For this review, take the finished solid that the model builds, in its own axes (mm). A direction names the side the tool comes from. Round coordinates to 2 decimals unless told otherwise and drop trailing zeros. Write each loop counter-clockwise with the first axis right and the second up, starting at its lowest first coordinate (ties: lowest second). Pieces come first, ordered by that corner, then holes. Notation, with made-up numbers: M 51.5,79 L 73.5,79 A18 ccw 73.5,110 Z; hole C 75,15 d2. An arc over 180 degrees is marked long. Write each question's results on one line, items separated by ' | '. Start each with the question number.
```python
from build123d import *

# Parameters (mm, degrees)
SKETCH1_W           = 32.6
SKETCH1_H           = 15.1
SKETCH1_R           = 1.5
BOSS_EXTRUDE1_DEPTH = 1.5
SKETCH2_W           = 40
SKETCH2_H           = 13.5
SKETCH2_R           = 1.5
BOSS_EXTRUDE2_DEPTH = 1.5
FILLET1_R           = 10
FILLET2_R           = 1


with BuildPart() as part:
    # Sketch1 → Boss-Extrude1 (new body)
    with BuildSketch(Plane.XY):
        Rectangle(SKETCH1_W, SKETCH1_H)
        with Locations((-14, 5.5)):
            Circle(SKETCH1_R, mode=Mode.SUBTRACT)
        with Locations((-14, -5.5)):
            Circle(SKETCH1_R, mode=Mode.SUBTRACT)
    extrude(amount=BOSS_EXTRUDE1_DEPTH)

    # Sketch2 → Boss-Extrude2 (add)
    with BuildSketch(Plane.XZ.offset(7.55)):
        with Locations((0, -5.25)):
            Rectangle(SKETCH2_W, SKETCH2_H)
        with Locations(Location((-15, -6, 0), (0, 0, 270))):
            Circle(SKETCH2_R, mode=Mode.SUBTRACT)
        with Locations(Location((15, -6, 0), (0, 0, 270))):
            Circle(SKETCH2_R, mode=Mode.SUBTRACT)
    extrude(amount=BOSS_EXTRUDE2_DEPTH)

    # Fillet1
    # the kernel refuses this fillet: 10 mm, written as the material it adds along each edge
    with BuildSketch(Plane(origin=(16.3, -7.55, 0), x_dir=(1, 0, 0), z_dir=(0, 0, 1))) as fillet1_piece_1:
        with BuildLine():
            CenterArc((10, 7.765951326), FILLET1_R, 180, 50.949877464)
            Line((0, 7.765951326), (-0.2, 7.765951326))
            Line((-0.2, 7.765951326), (-0.2, 0))
            Line((-0.2, 0), (0, -0.2))
            ThreePointArc((0, -0.2), (1.85, -0.2), (3.574, -0.155319027))
            Line((3.574, -0.155319027), (3.7, 0))
        make_face()
    extrude(amount=1.5)
    with BuildSketch(Plane(origin=(-16.3, -7.55, 0), x_dir=(-1, 0, 0), z_dir=(0, 0, 1))) as fillet1_piece_2:
        with BuildLine():
            CenterArc((10, -7.765951326), FILLET1_R, 129.050122536, 50.949877464)
            Line((0, -7.765951326), (-0.2, -7.765951326))
            Line((-0.2, -7.765951326), (-0.2, 0))
            Line((-0.2, 0), (0, 0.2))
            ThreePointArc((0, 0.2), (1.85, 0.2), (3.574, 0.155319027))
            Line((3.574, 0.155319027), (3.7, 0))
        make_face()
    extrude(amount=1.5)

    # Fillet2
    fillet2_edges = [part.edges().sort_by_distance(p)[0] for p in [
        (-20, -8.3, 1.5),
        (0, -7.55, -12),
        (-20, -8.3, -12),
        (20, -8.3, -12),
        (20, -8.3, 1.5),
        (-16.3, 7.55, 0.75),
        (16.3, 7.55, 0.75),
    ]]
    fillet(fillet2_edges, radius=FILLET2_R)


solid = part.part
```
Item 1: We need section D-D on x = -3.5. State the section outline as (y, z) points.
Item 2: For faces 5 (the flat face through (16.3, 3, 1)), 6 (the flat face through (0, -7.55, -5)), 7 (the flat face through (0, 7.55, 1)), 8 (the flat face through (-16.3, 3, 1)), 9 (the flat face through (-20, -8, -5)), list the 3-axis set-ups (+Z, -Z, +X, -X, +Y, -Y) from which the entire face can be reached by the end or side of a thin tool; tool diameter is ignored.
Item 3: We need section C-C on x = -14. State the section outline as (y, z) points, then the cut area to 3 significant figures.
Item 4: Insertion check: P1, Ø2.5, axis at x = 15, z = -6, coming from the -Y side; P2, Ø1.6, axis at y = 4, z = 1, coming from the -X side; P3, Ø1, axis at x = -16, y = -4, coming from the -Z side. Each pin has a flat end and moves straight along its axis. Give the tip position at first contact, or say it passes through.
Item 5: We need section B-B on z = -6. State the section outline as (x, y) points, then the cut area to 3 significant figures.
Item 6: We need section A-A on y = 5.5. State the section outline as (x, z) points.
Item 7: For probe 1 along Y at (x, z) = (-14, 0.9); probe 2 along X at (y, z) = (-8.3, -6); probe 3 along Z at (x, y) = (-17, -4), list the stretches that pass through material, from the lowest coordinate up.
Item 8: Mouldability with a two-part tool opening along Z and no side actions: class faces 1 (the flat face through (0, 0, 0)), 2 (the cylindrical face through (16.01, -8.29, -4.89)), 3 (the cylindrical face through (-14.93, -8.29, -4.5)), 4 (the cylindrical face through (-15.999, 7.265, 0.76)) as pulls with the +Z half, pulls with the -Z half, needs draft (parallel to the pull), parting line crosses it, or undercut.
Numbers:
1) outline: M -9.05,-12 L -8.55,-12 A1 ccw -7.55,-11 L -7.55,0 L 7.55,0 L 7.55,1.5 L -9.05,1.5 Z
2) face 5: +Z, -Z, +X, +Y | face 6: -Z, +X, -X, +Y | face 7: +Z, -Z, +X, -X, +Y | face 8: +Z, -Z, -X, +Y | face 9: +Z, -Z, -X, +Y, -Y
3) outline: M -9.05,-12 L -8.55,-12 A1 ccw -7.55,-11 L -7.55,-7.12 L -9.05,-7.12 Z; M -9.05,-4.88 L -7.55,-4.88 L -7.55,0 L -7,0 L -7,1.5 L -9.05,1.5 Z; M -4,0 L 4,0 L 4,1.5 L -4,1.5 Z; M 7,0 L 7.55,0 L 7.55,1.5 L 7,1.5 Z | area: 30.3 mm^2
4) P1: passes through | P2: stops at x = -16.3 | P3: stops at z = 0
5) outline: M -20,-9.05 L -16.5,-9.05 L -16.5,-7.55 L -20,-7.55 Z; M -13.5,-9.05 L 13.5,-9.05 L 13.5,-7.55 L -13.5,-7.55 Z; M 16.5,-9.05 L 20,-9.05 L 20,-7.55 L 16.5,-7.55 Z | area: 51.0 mm^2
6) outline: M -16.3,0 L -15.5,0 L -15.5,1.5 L -16.3,1.5 Z; M -12.5,0 L 16.3,0 L 16.3,1.5 L -12.5,1.5 Z
7) probe 1: y = -9.05 to -7, -4 to 4, 7 to 7.55 | probe 2: x = -20 to -16.5, -13.5 to 13.5, 16.5 to 20 | probe 3: z = 0 to 1.5
8) face 1: pulls with the -Z half | face 2: undercut | face 3: undercut | face 4: needs draft
